from build123d import *

# Parameters (mm, degrees)
SKETCH1_W                 = 10
SKETCH1_H                 = 10
F_40_X_40A_X_R0_5_1_DEPTH = 1030
SKETCH_2_R                = 2.5
CUT_EXTRUDE_1_DEPTH       = 1031.580050263


with BuildPart() as part:
    # Sketch1 → 铝型材 40 X 40A X R0.5(1) (new body)
    with BuildSketch(Plane.YX):
        with BuildLine():
            Line((-19.5, 20), (-4.5, 20))
            Line((-4.5, 20), (-4.5, 18.2))
            Line((-4.5, 18.2), (-7.1, 18.2))
            Line((-7.1, 18.2), (-7.1, 8.2))
            Line((-7.1, 8.2), (7.1, 8.2))
            Line((7.1, 8.2), (7.1, 18.2))
            Line((7.1, 18.2), (4.5, 18.2))
            Line((4.5, 18.2), (4.5, 20))
            Line((4.5, 20), (19.5, 20))
            ThreePointArc((19.5, 20), (19.853553391, 19.853553391), (20, 19.5))
            Line((20, 19.5), (20, 4.5))
            Line((20, 4.5), (18.2, 4.5))
            Line((18.2, 4.5), (18.2, 7.1))
            Line((18.2, 7.1), (8.2, 7.1))
            Line((8.2, 7.1), (8.2, -7.1))
            Line((8.2, -7.1), (18.2, -7.1))
            Line((18.2, -7.1), (18.2, -4.5))
            Line((18.2, -4.5), (20, -4.5))
            Line((20, -4.5), (20, -19.5))
            ThreePointArc((20, -19.5), (19.853553391, -19.853553391), (19.5, -20))
            Line((19.5, -20), (4.5, -20))
            Line((4.5, -20), (4.5, -18.2))
            Line((4.5, -18.2), (7.1, -18.2))
            Line((7.1, -18.2), (7.1, -8.2))
            Line((7.1, -8.2), (-7.1, -8.2))
            Line((-7.1, -8.2), (-7.1, -18.2))
            Line((-7.1, -18.2), (-4.5, -18.2))
            Line((-4.5, -18.2), (-4.5, -20))
            Line((-4.5, -20), (-19.5, -20))
            ThreePointArc((-19.5, -20), (-19.853553391, -19.853553391), (-20, -19.5))
            Line((-20, -19.5), (-20, -4.5))
            Line((-20, -4.5), (-18.2, -4.5))
            Line((-18.2, -4.5), (-18.2, -7.1))
            Line((-18.2, -7.1), (-8.2, -7.1))
            Line((-8.2, -7.1), (-8.2, 7.1))
            Line((-8.2, 7.1), (-18.2, 7.1))
            Line((-18.2, 7.1), (-18.2, 4.5))
            Line((-18.2, 4.5), (-20, 4.5))
            Line((-20, 4.5), (-20, 19.5))
            ThreePointArc((-20, 19.5), (-19.853553391, 19.853553391), (-19.5, 20))
        make_face()
        with BuildLine():
            Line((-4.87903679, 6.434671709), (-4.110433762, 5.66606868))
            ThreePointArc((-4.110433762, 5.66606868), (0, 7), (4.110433762, 5.66606868))
            Line((4.110433762, 5.66606868), (4.87903679, 6.434671709))
            ThreePointArc((4.87903679, 6.434671709), (6.434671709, 6.434671709), (6.434671709, 4.87903679))
            Line((6.434671709, 4.87903679), (5.66606868, 4.110433762))
            ThreePointArc((5.66606868, 4.110433762), (7, 0), (5.66606868, -4.110433762))
            Line((5.66606868, -4.110433762), (6.434671709, -4.87903679))
            ThreePointArc((6.434671709, -4.87903679), (6.434671709, -6.434671709), (4.87903679, -6.434671709))
            Line((4.87903679, -6.434671709), (4.110433762, -5.66606868))
            ThreePointArc((4.110433762, -5.66606868), (0, -7), (-4.110433762, -5.66606868))
            Line((-4.110433762, -5.66606868), (-4.87903679, -6.434671709))
            ThreePointArc((-4.87903679, -6.434671709), (-6.434671709, -6.434671709), (-6.434671709, -4.87903679))
            Line((-6.434671709, -4.87903679), (-5.66606868, -4.110433762))
            ThreePointArc((-5.66606868, -4.110433762), (-7, 0), (-5.66606868, 4.110433762))
            Line((-5.66606868, 4.110433762), (-6.434671709, 4.87903679))
            ThreePointArc((-6.434671709, 4.87903679), (-6.434671709, 6.434671709), (-4.87903679, 6.434671709))
        make_face(mode=Mode.SUBTRACT)
        with Locations((-13.7, 13.7)):
            Rectangle(SKETCH1_W, SKETCH1_H, mode=Mode.SUBTRACT)
        with Locations((13.7, 13.7)):
            Rectangle(SKETCH1_W, SKETCH1_H, mode=Mode.SUBTRACT)
        with Locations((13.7, -13.7)):
            Rectangle(SKETCH1_W, SKETCH1_H, mode=Mode.SUBTRACT)
        with Locations((-13.7, -13.7)):
            Rectangle(SKETCH1_W, SKETCH1_H, mode=Mode.SUBTRACT)
    extrude(amount=F_40_X_40A_X_R0_5_1_DEPTH)

    # 草图2 → 切除-拉伸1 (cut, through all)
    with BuildSketch(Plane(origin=(8.2, 0, 0), x_dir=(0, 0, -1), z_dir=(1, 0, 0))):
        with Locations((40, 0)):
            Circle(SKETCH_2_R)
    extrude(amount=-CUT_EXTRUDE_1_DEPTH, mode=Mode.SUBTRACT)


solid = part.part
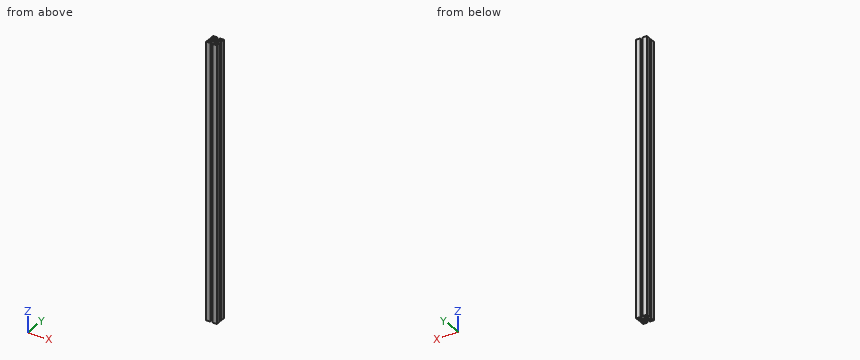
Source: CAD feature listing. Evaluate the final solid. Frame: model axes, mm. Give positions to 0.01 mm unless a question says otherwise; leave off trailing zeros. Answer as a JSON object with one key per item and string values.
Q1. Ray query, line 1 along X through (y, z) = (18.5, -764); line 2 along Y through (x, z) = (12, -577). Return the intervals inside material, ascending.
Geometry check:
{"line 1": "x = -20 to -18.7, -8.7 to -4.5, 4.5 to 8.7, 18.7 to 20", "line 2": "y = -20 to -18.7, -8.7 to -7.1, 7.1 to 8.7, 18.7 to 20"}
Q2. Contact query for flat-ended pins moving along their axis: P1, Ø2, axis at x = 1, z = -313, coming from the +Y side; P2, Ø6, axis at x = -1, y = -3, coming from the +Z side; P3, Ø3, axis at x = 9, y = -14, coming from the +Z side. Output: stop coordinate, or through.
Geometry check:
{"P1": "stops at y = 8.2", "P2": "passes through", "P3": "stops at z = 0"}
Q3. Cut plane A-A, the plane z = -116. Count the separate pieces of the cut face and the enclosed holes in it, then the cut area to 3 significant figures.
Geometry check:
{"separate pieces": "1", "enclosed holes": "5", "area": "396 mm^2"}
